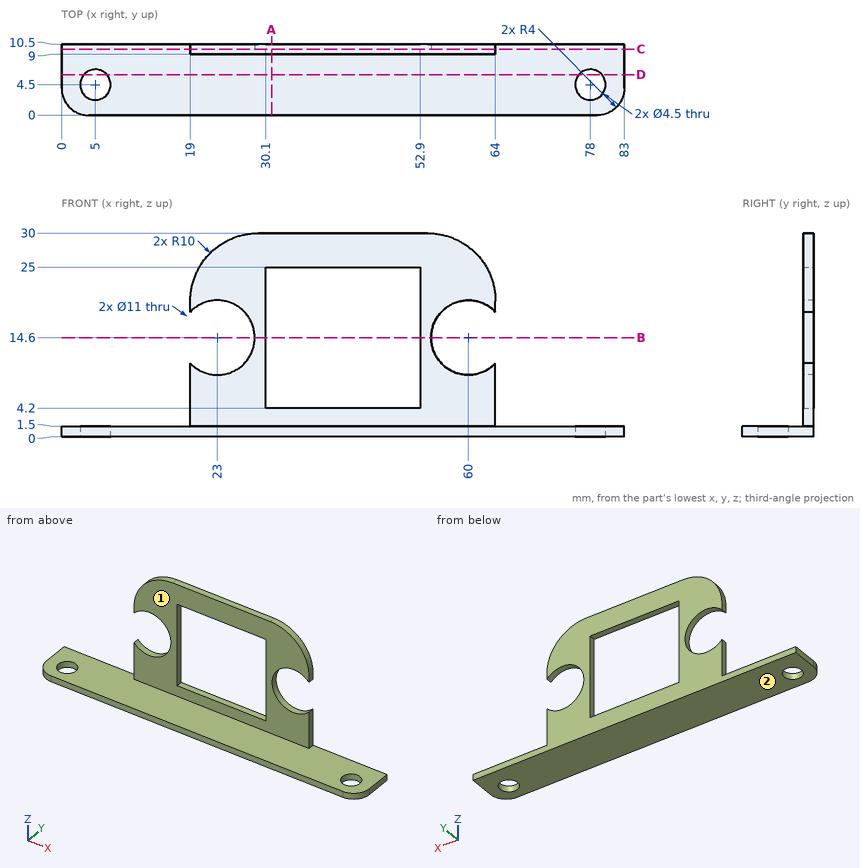
Check sheet for the drawn part. Datum: minimum x, y, z corner. Units: mm. A direction names the side the tool comes from. Coordinates: 2 decimals unless noted, no trailing zeros. Order: outer loops, then holes, each group sorted by start corner. A loop starts at its lowest first (then second) coordinate and runs counter-clockwise, first axis right, second up. Notation, with made-up numbers: M -20.75,4 L -7.75,4 A23 cw -7.75,31 Z; hole C 5,21.5 d10. An arc over 180 degrees is marked long. One line per item, written item: value. Start each with the question number.
Item 1: Access from +Z, -Z, +X, -X, +Y, -Y to the whole of each face (thin tool, end or side, straight path). Record for the marked faces 1 and 2.
Item 2: Sectioned sample at D-D (y = 6). Enter the section's corners in (x, z).
Item 3: Sectioned sample at C-C (y = 9.75). Enter the section's corners in (x, z).
Item 4: Sectioned sample at B-B (z = 14.6). Enter the section's corners in (x, y), then the cut area to 3 significant figures.
Item 5: Gauge pin test, flat ends, axial feed: pin 1 (0.8 mm diameter, centred on y = 9.5, z = 19.5, fed in from +X); pin 2 (10 mm diameter, centred on x = 20, z = 5.5, fed in from -Y); pin 3 (3 mm diameter, centred on x = 48, y = 4.5, fed in from +Z); pin 4 (10 mm diameter, centred on x = 23, z = 14.6, fed in from +Y). Record the tip position at first contact, or that the pin passes through.
Item 6: Sectioned sample at A-A (x = 31). Enter the section's corners in (y, z).
Item 7: Scan lines: probe 1 along Y at (x, z) = (5, 0.75); probe 2 along Z at (x, y) = (71, 9); probe 3 along Y at (x, z) = (34.5, 3). Record each from-to range of solid material in increasing order.
Conclusion:
1. face 1: +Z, +X, -X, -Y
1. face 2: -Z, +X, -X, +Y, -Y
2. outline: M 0,0 L 3.32,0 L 3.32,1.5 L 0,1.5 Z; M 6.68,0 L 76.32,0 L 76.32,1.5 L 6.68,1.5 Z; M 79.68,0 L 83,0 L 83,1.5 L 79.68,1.5 Z
3. outline: M 0,0 L 83,0 L 83,1.5 L 64,1.5 L 64,10.83 A5.5 cw long 64,18.37 L 64,20 A10 ccw 54,30 L 29,30 A10 ccw 19,20 L 19,18.37 A5.5 cw long 19,10.83 L 19,1.5 L 0,1.5 Z; hole M 30.1,4.2 L 52.9,4.2 L 52.9,25 L 30.1,25 Z
4. outline: M 28.5,9 L 30.1,9 L 30.1,10.5 L 28.5,10.5 Z; M 52.9,9 L 54.5,9 L 54.5,10.5 L 52.9,10.5 Z
4. area: 4.80 mm^2
5. pin 1: stops at x = 64
5. pin 2: stops at y = 0
5. pin 3: stops at z = 1.5
5. pin 4: passes through
6. outline: M 0,0 L 10.5,0 L 10.5,4.2 L 9,4.2 L 9,1.5 L 0,1.5 Z; M 9,25 L 10.5,25 L 10.5,30 L 9,30 Z
7. probe 1: y = 0 to 2.25, 6.75 to 10.5
7. probe 2: z = 0 to 1.5
7. probe 3: y = 9 to 10.5
